from build123d import *

# Parameters (mm, degrees)
SKETCH_1_W          = 10
SKETCH_1_H          = 2
EXTRUDE_1_DEPTH     = 395
SKETCH_2_R          = 0.8
SKETCH_2_W          = 4
SKETCH_2_H          = 2
CUT_EXTRUDE_1_DEPTH = 1168.361381654


with BuildPart() as part:
    # 草图1 → 凸台-拉伸1 (new body)
    with BuildSketch(Plane.XY.offset(1160.01)):
        with Locations((125.787596038, -4.389694097)):
            Rectangle(SKETCH_1_W, SKETCH_1_H)
    extrude(amount=-EXTRUDE_1_DEPTH)

    # 草图2 → 切除-拉伸1 (cut, through all)
    with BuildSketch(Plane(origin=(0, -3.389694097, 0), x_dir=(1, 0, 0), z_dir=(0, 1, 0))):
        with Locations(Location((127.787596038, -772.51, 0), (0, 0, 180))):
            Circle(SKETCH_2_R)
        with Locations(Location((127.787596038, -778.51, 0), (0, 0, 180))):
            Circle(SKETCH_2_R)
        with Locations(Location((127.787596038, -940.51, 0), (0, 0, 180))):
            Circle(SKETCH_2_R)
        with Locations(Location((127.787596038, -946.51, 0), (0, 0, 180))):
            Circle(SKETCH_2_R)
        with Locations(Location((127.787596038, -1041.51, 0), (0, 0, 180))):
            Circle(SKETCH_2_R)
        with Locations(Location((127.787596038, -1035.51, 0), (0, 0, 180))):
            Circle(SKETCH_2_R)
        with Locations((122.787596038, -891.01)):
            Rectangle(SKETCH_2_W, SKETCH_2_H)
        with Locations((122.787596038, -766.01)):
            Rectangle(SKETCH_2_W, SKETCH_2_H)
        with Locations((122.787596038, -1016.01)):
            Rectangle(SKETCH_2_W, SKETCH_2_H)
        with Locations((122.787596038, -1141.01)):
            Rectangle(SKETCH_2_W, SKETCH_2_H)
        with Locations((122.787596038, -1159.01)):
            Rectangle(SKETCH_2_W, SKETCH_2_H)
    extrude(amount=-CUT_EXTRUDE_1_DEPTH, mode=Mode.SUBTRACT)


solid = part.part
The model under review builds one solid part; all positions refer to its coordinate system, in mm. Coordinates: 2 decimals unless noted, no trailing zeros. Order: outer loops, then holes, each group sorted by start corner. A loop starts at its lowest first (then second) coordinate and runs counter-clockwise, first axis right, second up. Notation, with made-up numbers: (47, -33.75) -> (82, -33.75) arc R33 ccw to (82, 5.25) -> close; hole circle Ø2 at (-5, 33). An arc over 180 degrees is marked (long way). Answer in a Markdown table with one row per item.
(1) Wall thickness on line 1 along Z through (x, y) = (123, -5); line 2 along X through (y, z) = (-4, 778.51): over which ranges is each line inside the solid? List them lowest first.
Answers:
| item | result |
|---|---|
| line 1 | 767.01 to 890.01, 892.01 to 1015.01, 1017.01 to 1140.01, 1142.01 to 1158.01 |
| line 2 | 120.79 to 126.99, 128.59 to 130.79 |
(2) Consider section A-A (x = 123.25). Write out the cut boundary in (y, z).
Answers:
| item | result |
|---|---|
| outline | (-5.39, 767.01) -> (-3.39, 767.01) -> (-3.39, 890.01) -> (-5.39, 890.01) -> close; (-5.39, 892.01) -> (-3.39, 892.01) -> (-3.39, 1015.01) -> (-5.39, 1015.01) -> close; (-5.39, 1017.01) -> (-3.39, 1017.01) -> (-3.39, 1140.01) -> (-5.39, 1140.01) -> close; (-5.39, 1142.01) -> (-3.39, 1142.01) -> (-3.39, 1158.01) -> (-5.39, 1158.01) -> close |
(3) Insertion check: pin 1 (0.6 mm diameter, centred on x = 123, y = -4.5, fed in from -Z); pin 2 (1 mm diameter, centred on x = 123, y = -4.5, fed in from +Z); pin 3 (1 mm diameter, centred on y = -4.5, z = 1016, fed in from -X). Each pin has a flat end and moves straight along its axis. Give the tip position at first contact, or say it passes through.
Answers:
| item | result |
|---|---|
| pin 1 | z = 767.01 |
| pin 2 | z = 1158.01 |
| pin 3 | x = 124.79 |
